Work out the finished part from the listing and answer in its coordinate system (mm). A direction names the side the tool comes from. Round coordinates to 2 decimals unless told otherwise and drop trailing zeros. Return JSON: item names as keys, results as strings.
from build123d import *

# Parameters (mm, degrees)
F1_DEPTH = 76.2
F2_R     = 5.08
F3_SIZE  = 5.08


with BuildPart() as f1:
    # F0 (on Front) → F1 (new body)
    with BuildSketch(Plane.XZ):
        Polygon((0, 76.605852), (-76.198919, 76.2), (-76.198919, 0), (0, 0), align=None)
    extrude(amount=F1_DEPTH)

    # F2
    f2_edges = [f1.edges().sort_by_distance(p)[0] for p in [
        (-38.09946, 0, 76.402926),
        (-76.198919, -38.1, 76.2),
        (0, -38.1, 76.605852),
        (-38.09946, -76.2, 76.402926),
    ]]
    fillet(f2_edges, radius=F2_R)

    # F3
    f3_edges = [f1.edges().sort_by_distance(p)[0] for p in [
        (-76.198919, -38.1, 0),
        (-38.09946, -76.2, 0),
        (0, -38.1, 0),
        (-38.09946, 0, 0),
    ]]
    chamfer(f3_edges, length=F3_SIZE)


solid = f1.part
Item 1: Consider line 1 along Z through (x, y) = (-6.5, -10); line 2 along Z through (x, y) = (-65, -59); line 3 along Y through (x, z) = (-34.5, 4.5). Determine where each line is inside the solid, lowest interval first. Write a range as [from, to].
Output:
{"line 1": "z = [0, 76.57]", "line 2": "z = [0, 76.26]", "line 3": "y = [-75.62, -0.58]"}
Item 2: This flat-tipped pin is pushed along its axis until it touches: pin 1 (3 mm diameter, centred on x = -51.5, y = -23, fed in from +Z). Where does it stop, or does it pass through?
Output:
{"pin 1": "stops at z = 76.34"}
Item 3: Which of the six approach directions +Z, -Z, +X, -X, +Y, -Y give full straight-line access (tool end or side, diameter ignored) to faces 1 (the cylindrical face through (-38.652, -74.672, 74.951)), 2 (the flat face through (-76.199, -38, 39)), 3 (the cylindrical face through (-38.652, -1.528, 74.951))?
Output:
{"face 1": "+Z, -X, -Y", "face 2": "+Z, -Z, -X, +Y, -Y", "face 3": "+Z, -X, +Y"}
